from build123d import *

# Parameters (mm, degrees)
SKETCH_1_W                  = 20
SKETCH_1_H                  = 20
SKETCH_1_W_2                = 17
SKETCH_1_H_2                = 17
EXTRUDE_1_DEPTH             = 620
SKETCH_2_R                  = 2.7
CUT_EXTRUDE_1_DEPTH         = 25
SKETCH_3_R                  = 2.25
CUT_EXTRUDE_2_DEPTH         = 25
SKETCH_4_R                  = 2.7
CUT_EXTRUDE_3_DEPTH         = 40
SKETCH_6_R                  = 5
CUT_EXTRUDE_4_DEPTH         = 10
CUT_EXTRUDE_START           = 10
SKETCH_7_R                  = 5
CUT_EXTRUDE_5_DEPTH         = 20
CUT_EXTRUDE_START_2         = -10
SKETCH_8_R                  = 5
CUT_EXTRUDE_6_DEPTH         = 30
SKETCH_9_R                  = 5
CUT_EXTRUDE_7_DEPTH         = 5
HOLE_WIZARD_4_3_4_3_1_D     = 4.3
HOLE_WIZARD_10_0_10_1_D     = 10
HOLE_WIZARD_10_0_10_1_DEPTH = 1.5


with BuildPart() as part:
    # ｽｹｯﾁ1 → ﾎﾞｽ - 押し出し1 (new body)
    with BuildSketch(Plane.XY):
        Rectangle(SKETCH_1_W, SKETCH_1_H)
        Rectangle(SKETCH_1_W_2, SKETCH_1_H_2, mode=Mode.SUBTRACT)
    extrude(amount=EXTRUDE_1_DEPTH)

    # ｽｹｯﾁ2 → ｶｯﾄ - 押し出し1 (cut)
    with BuildSketch(Plane(origin=(10, 0, 0), x_dir=(0, 0, -1), z_dir=(1, 0, 0))):
        with Locations((-585, 0)):
            Circle(SKETCH_2_R)
        with Locations((-35, 0)):
            Circle(SKETCH_2_R)
        with Locations((-335, 0)):
            Circle(SKETCH_2_R)
    extrude(amount=-CUT_EXTRUDE_1_DEPTH, mode=Mode.SUBTRACT)

    # ｽｹｯﾁ3 → ｶｯﾄ - 押し出し2 (cut)
    with BuildSketch(Plane(origin=(0, 10, 0), x_dir=(1, 0, 0), z_dir=(0, 1, 0))):
        with Locations((0, -22)):
            Circle(SKETCH_3_R)
        with Locations((0, -610)):
            Circle(SKETCH_3_R)
        with Locations((0, -530)):
            Circle(SKETCH_3_R)
        with Locations((0, -590)):
            Circle(SKETCH_3_R)
    extrude(amount=-CUT_EXTRUDE_2_DEPTH, mode=Mode.SUBTRACT)

    # ｽｹｯﾁ4 → ｶｯﾄ - 押し出し3 (cut)
    with BuildSketch(Plane(origin=(10, 0, 0), x_dir=(0, 0, -1), z_dir=(1, 0, 0))):
        with Locations((-15, 0)):
            Circle(SKETCH_4_R)
        with Locations((-5, 0)):
            Circle(SKETCH_4_R)
        with Locations((-615, 0)):
            Circle(SKETCH_4_R)
        with Locations((-605, 0)):
            Circle(SKETCH_4_R)
    extrude(amount=-CUT_EXTRUDE_3_DEPTH, mode=Mode.SUBTRACT)

    # ｽｹｯﾁ6 → ｶｯﾄ - 押し出し4 (cut)
    with BuildSketch(Plane(origin=(0, -10, 0), x_dir=(-1, 0, 0), z_dir=(0, -1, 0))):
        with Locations((0, -530)):
            Circle(SKETCH_6_R)
    extrude(amount=-CUT_EXTRUDE_4_DEPTH, mode=Mode.SUBTRACT)

    # ｽｹｯﾁ7 → ｶｯﾄ - 押し出し5 (cut)
    with BuildSketch(Plane(origin=(-10, 0, 0), x_dir=(0, 0, -1), z_dir=(1, 0, 0)).offset(CUT_EXTRUDE_START)):
        with Locations((-585, 0)):
            Circle(SKETCH_7_R)
        with Locations((-335, 0)):
            Circle(SKETCH_7_R)
        with Locations((-35, 0)):
            Circle(SKETCH_7_R)
    extrude(amount=CUT_EXTRUDE_5_DEPTH, mode=Mode.SUBTRACT)

    # ｽｹｯﾁ8 → ｶｯﾄ - 押し出し6 (cut)
    with BuildSketch(Plane(origin=(10, 0, 0), x_dir=(0, 0, -1), z_dir=(1, 0, 0)).offset(CUT_EXTRUDE_START_2)):
        with Locations((-605, 0)):
            Circle(SKETCH_8_R)
    extrude(amount=-CUT_EXTRUDE_6_DEPTH, mode=Mode.SUBTRACT)

    # ｽｹｯﾁ9 → ｶｯﾄ - 押し出し7 (cut)
    with BuildSketch(Plane.ZY.offset(10)):
        with Locations((15, 0)):
            Circle(SKETCH_9_R)
    extrude(amount=-CUT_EXTRUDE_7_DEPTH, mode=Mode.SUBTRACT)

    # Ø4.3 (4.3) 直径の穴1 (through all)
    with Locations(Plane(origin=(10, 0, 0), x_dir=(0, 0, -1), z_dir=(1, 0, 0))):
        with Locations((-460, 0), (-310, 0), (-160, 0)):
            Hole(HOLE_WIZARD_4_3_4_3_1_D / 2)

    # Ø10.0 (10) 直径の穴1
    with Locations(Plane.ZY.offset(10)):
        with Locations((160, 0), (310, 0), (460, 0)):
            Hole(HOLE_WIZARD_10_0_10_1_D / 2, depth=HOLE_WIZARD_10_0_10_1_DEPTH)


solid = part.part
The model under review builds one solid part; all positions refer to its coordinate system, in mm. A direction names the side the tool comes from. Round coordinates to 2 decimals unless told otherwise and drop trailing zeros. Order: outer loops, then holes, each group sorted by start corner. A loop starts at its lowest first (then second) coordinate and runs counter-clockwise, first axis right, second up. Notation, with made-up numbers: (-37.75, 60.25) -> (14.25, 60.25) arc R26 ccw to (14.25, 76.25) -> close; hole circle Ø9 at (11, -9.5). An arc over 180 degrees is marked (long way). Return JSON: item names as keys, results as strings.
1. Take a section at A-A (z = 79.5). Write out the cut boundary in (x, y).
Answer block:
{"outline": "(-10, -10) -> (10, -10) -> (10, 10) -> (-10, 10) -> close; hole (-8.5, -8.5) -> (8.5, -8.5) -> (8.5, 8.5) -> (-8.5, 8.5) -> close"}
2. The part is to be moulded in two halves that separate along Z. For faces 4 (the face through (9.24, 1.5, 330.23)), 5 (the face through (-9, 0, 620)), 6 (the face through (0, -8.5, 306)), say which applies: +Z half, -Z half, draft (parallel to the pull), parting line (faces both ways), or undercut.
Answer block:
{"face 4": "undercut", "face 5": "+Z half", "face 6": "draft"}
3. For faces 1 (the face through (9, 0, 40)), 2 (the face through (0.651, -9.26, 525.043)), 3 (the face through (-9.24, 1.5, 305.23)), list the 3-axis set-ups (+Z, -Z, +X, -X, +Y, -Y) from which the entire face can be reached by the end or side of a thin tool; tool diameter is ignored.
Answer block:
{"face 1": "+X", "face 2": "-Y", "face 3": "-X"}
4. Insertion check: P1, Ø5, axis at x = 0, z = 610, coming from the +Y side; P2, Ø8, axis at y = 0, z = 160, coming from the -X side; P3, Ø8.5, axis at y = 0, z = 35, coming from the +X side. Each pin has a flat end and moves straight along its axis. Give the tip position at first contact, or say it passes through.
Answer block:
{"P1": "stops at y = 10", "P2": "stops at x = 8.5", "P3": "stops at x = -8.5"}
5. For L1, parallel to Z at x = 0, y = -9.05; L2, parallel to Y at x = 9, z = 585; L3, parallel to X at y = -6, z = 210.5, list the stretches that pass through material, from the lowest coordinate up. Write a range as [from, to].
Answer block:
{"L1": "z = [0, 19.75], [24.25, 525], [535, 587.75], [592.25, 607.75], [612.25, 620]", "L2": "y = [-10, -5], [5, 10]", "L3": "x = [-10, -8.5], [8.5, 10]"}
